Design review of the part shown in the three views and the two pictorial views. Dimensions are in mm from the part's minimum x, y and z. Round coordinates to 2 decimals unless told otherwise and drop trailing zeros. Order: outer loops, then holes, each group sorted by start corner. A loop starts at its lowest first (then second) coordinate and runs counter-clockwise, first axis right, second up. Notation, with made-up numbers: M 21.25,-17 L 48.25,-17 A8 ccw 48.25,-13 Z; hole C 34.25,77 d2. An arc over 180 degrees is marked long. Write each question's results on one line, items separated by ' | '. Start each with the question number.
Item 1: Take a section at C-C, the plane z = 1.75. Write out the cut boundary in (x, y), plus the area to 3 significant figures.
Item 2: The part is to be moulded in two halves that separate along X. For the marked faces 1, 2 and 3, say which applies: +X half, -X half, draft (parallel to the pull), parting line (faces both ways), or undercut.
Item 3: Clearance check with flat-ended pins moving along their axes: pin 1 (5 mm diameter, centred on y = 5, z = 6.5, fed in from +X); pin 2 (4 mm diameter, centred on y = 9, z = 11, fed in from +X); pin 3 (1.5 mm diameter, centred on x = 1.5, z = 2, fed in from -Y) (1 decimal); pin 4 (3.5 mm diameter, centred on x = 5.4, y = 5.4, fed in from -Z). State where each tip first meets the part, or that it passes through.
Item 4: Take a section at D-D, the plane y = 8. Write out the cut boundary in (x, z) (1 decimal).
Item 5: Take a section at A-A, the plane y = 5.4. Write out the cut boundary in (x, z).
Item 6: Wall thickness on line 1 (Y direction, x = 5.4, z = 1.85); line 2 (Y direction, x = 5.4, z = 6.5); line 3 (X direction, y = 6.75, z = 6): over which ranges is each line inside the solid? List them lowest first. Write a range as [from, to].
Item 7: Take a section at B-B, the plane x = 5.4. Write out the cut boundary in (y, z).
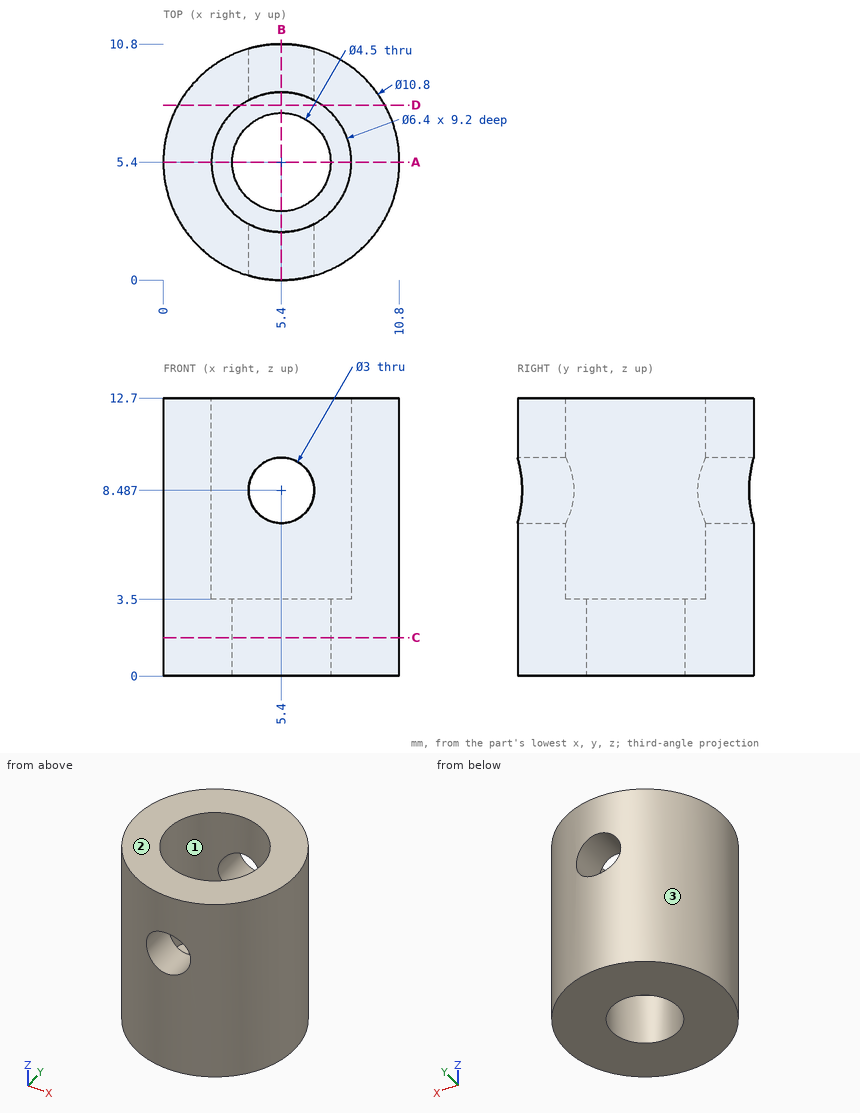
Results list:
1) outline: C 5.4,5.4 d10.8; hole C 5.4,5.4 d4.5 | area: 75.7 mm²
2) face 1: undercut | face 2: draft | face 3: parting line
3) pin 1: x = 10.8 | pin 2: x = 10.56 | pin 3: y = 1 | pin 4: through
4) outline: M 0.7,0 L 10.1,0 L 10.1,12.7 L 7.3,12.7 L 7.3,3.5 L 3.5,3.5 L 3.5,12.7 L 0.7,12.7 Z
5) outline: M 0,0 L 3.15,0 L 3.15,3.5 L 2.2,3.5 L 2.2,12.7 L 0,12.7 Z; M 7.65,0 L 10.8,0 L 10.8,12.7 L 8.6,12.7 L 8.6,3.5 L 7.65,3.5 Z
6) line 1: [0, 3.15], [7.65, 10.8] | line 2: [0, 2.2], [8.6, 10.8] | line 3: [0.17, 2.5], [8.3, 10.63]
7) outline: M 0,0 L 3.15,0 L 3.15,3.5 L 2.2,3.5 L 2.2,6.99 L 0,6.99 Z; M 0,9.99 L 2.2,9.99 L 2.2,12.7 L 0,12.7 Z; M 7.65,0 L 10.8,0 L 10.8,6.99 L 8.6,6.99 L 8.6,3.5 L 7.65,3.5 Z; M 8.6,9.99 L 10.8,9.99 L 10.8,12.7 L 8.6,12.7 Z
